The listing builds one solid part. Answer for the finished solid, in the listing's coordinates (mm). Face numbers are marked on the shaded views. A direction names the side the tool comes from. Round coordinates to 2 decimals unless told otherwise and drop trailing zeros. Write item = value, one per line.
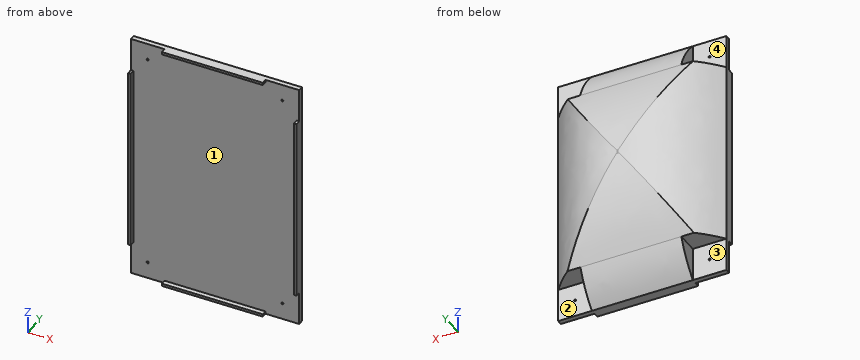
from build123d import *

# Parameters (mm, degrees)
CROQUIS1_W                = 100
CROQUIS1_H                = 150
SALIENTE_EXTRUIR1_DEPTH   = 30
CROQUIS3_W                = 1.5
CROQUIS3_H                = 110
CROQUIS3_W_2              = 60
CROQUIS3_H_2              = 1.5
SALIENTE_EXTRUIR2_DEPTH   = 3
CROQUIS5_W                = 20
CROQUIS5_H                = 20
CORTAR_EXTRUIR2_DEPTH     = 27
CROQUIS6_R                = 0.6
CORTAR_EXTRUIR3_DEPTH     = 95.09569597
SIMETR_A2_COPY_1_SKETCH_R = 0.6
SIMETR_A2_COPY_1_DEPTH    = 95.09569597
CORTAR_EXTRUIR4_DEPTH     = 129.549601322
CORTAR_EXTRUIR5_START     = -150
CORTAR_EXTRUIR5_DEPTH     = 150
CORTAR_EXTRUIR6_DEPTH     = 114.688170172
CORTAR_EXTRUIR7_DEPTH     = 114.688170172


# Read off the part's stored shape, not the designer's step: Cortar-Extruir5
with BuildPart() as part:
    # Croquis1 → Saliente-Extruir1 (new body)
    with BuildSketch(Plane(origin=(0, 0, 0), x_dir=(1, 0, 0), z_dir=(0, 1, 0))):
        Rectangle(CROQUIS1_W, CROQUIS1_H)
    extrude(amount=SALIENTE_EXTRUIR1_DEPTH)

    # Croquis3 → Saliente-Extruir2 (add)
    with BuildSketch(Plane.XZ):
        with Locations((-49.25, 0)):
            Rectangle(CROQUIS3_W, CROQUIS3_H)
        with Locations((0, -74.25)):
            Rectangle(CROQUIS3_W_2, CROQUIS3_H_2)
        with Locations((49.25, 0)):
            Rectangle(CROQUIS3_W, CROQUIS3_H)
        with Locations((0, 74.25)):
            Rectangle(CROQUIS3_W_2, CROQUIS3_H_2)
    extrude(amount=SALIENTE_EXTRUIR2_DEPTH)

    # Croquis5 → Cortar-Extruir2 (cut)
    with BuildSketch(Plane(origin=(0, 30, 0), x_dir=(1, 0, 0), z_dir=(0, 1, 0))):
        with Locations((-40, 65)):
            Rectangle(CROQUIS5_W, CROQUIS5_H)
        with Locations((40, 65)):
            Rectangle(CROQUIS5_W, CROQUIS5_H)
        with Locations((40, -65)):
            Rectangle(CROQUIS5_W, CROQUIS5_H)
        with Locations((-40, -65)):
            Rectangle(CROQUIS5_W, CROQUIS5_H)
    extrude(amount=-CORTAR_EXTRUIR2_DEPTH, mode=Mode.SUBTRACT)

    # Croquis6 → Cortar-Extruir3 (cut, through all)
    with BuildSketch(Plane(origin=(0, 3, 0), x_dir=(1, 0, 0), z_dir=(0, 1, 0))):
        with Locations(Location((40, 65, 0), (0, 0, 270))):
            Circle(CROQUIS6_R)
    cortar_extruir3 = extrude(amount=-CORTAR_EXTRUIR3_DEPTH, mode=Mode.SUBTRACT)

    # Simetría1: Cortar-Extruir3 across plane
    add(cortar_extruir3.mirror(Plane.XY), mode=Mode.SUBTRACT)

    # Simetría2: Cortar-Extruir3 across plane
    add(cortar_extruir3.mirror(Plane(origin=(0, 0, 0), x_dir=(0, 0, 1), z_dir=(1, 0, 0))), mode=Mode.SUBTRACT)

    # Simetría2 copy 1 sketch → Simetría2 copy 1 (cut, through all)
    with BuildSketch(Plane(origin=(0, 3, 0), x_dir=(-1, 0, 0), z_dir=(0, 1, 0))):
        with Locations(Location((40, 65, 0), (0, 0, 270))):
            Circle(SIMETR_A2_COPY_1_SKETCH_R)
    extrude(amount=-SIMETR_A2_COPY_1_DEPTH, mode=Mode.SUBTRACT)

    # Croquis7 → Cortar-Extruir4 (cut, through all)
    with BuildSketch(Plane.ZY.offset(50)):
        with BuildLine():
            Line((-55, 30), (-55, 15.839120061))
            add(Edge.make_bspline(
                [(-55, 15.839120061), (-28.872240535, 29.681618902), (-0.383648773, 29.996375418)],
                knots=[0.272557177, 0.272557177, 0.272557177, 0.972153635, 0.972153635, 0.972153635], degree=2))
            add(Edge.make_bspline(
                [(-0.015370594, 30), (-0.199457484, 29.998481088), (-0.383648773, 29.996375418)],
                knots=[0.9954153, 0.9954153, 0.9954153, 1, 1, 1], degree=2))
            Line((-0.015370594, 30), (-55, 30))
        make_face()
        with BuildLine():
            Line((55, 30), (1.887981045, 30))
            add(Edge.make_bspline(
                [(55, 16.129627481), (29.637077968, 29.770366226), (1.887981045, 30)],
                knots=[0.278550096, 0.278550096, 0.278550096, 0.971678885, 0.971678885, 0.971678885], degree=2))
            Line((55, 16.129627481), (55, 30))
        make_face()
    extrude(amount=-CORTAR_EXTRUIR4_DEPTH, mode=Mode.SUBTRACT)

    # Cortar-Extruir5 outline → Cortar-Extruir5 (cut)
    with BuildSketch(Plane.XY.offset(75).offset(CORTAR_EXTRUIR5_START)):
        with BuildLine():
            Line((7.5e-08, 30.000000001), (-50, 30))
            Line((-50, 30), (-50, 3))
            add(Edge.make_bspline(
                [(-50, 3), (-28.36157969, 29.799939616), (7.5e-08, 30.000000001)],
                knots=[0, 0, 0, 0.985180711, 0.985180711, 0.985180711], degree=2))
        make_face()
        with BuildLine():
            Line((50, 3), (50, 30))
            Line((50, 30), (0.854762637, 30))
            add(Edge.make_bspline(
                [(0.854762637, 30), (28.715142785, 29.789747772), (50, 3)],
                knots=[0.41802479, 0.41802479, 0.41802479, 1.368246178, 1.368246178, 1.368246178], degree=2))
        make_face()
    extrude(amount=CORTAR_EXTRUIR5_DEPTH, mode=Mode.SUBTRACT)

    # Croquis10 → Cortar-Extruir6 (cut, through all)
    with BuildSketch(Plane.ZY.offset(30)):
        with BuildLine():
            Line((75, 3), (75, 42.786726144))
            Line((75, 42.786726144), (55, 42.786726144))
            Line((55, 42.786726144), (55, 16.107425877))
            add(Edge.make_bspline(
                [(75, 3), (66.353698685, 12.015089749), (55, 16.107425877)],
                knots=[0, 0, 0, 1, 1, 1], degree=2))
        make_face()
    extrude(amount=-CORTAR_EXTRUIR6_DEPTH, mode=Mode.SUBTRACT)

    # Croquis11 → Cortar-Extruir7 (cut, through all)
    with BuildSketch(Plane.ZY.offset(30)):
        with BuildLine():
            Line((-75, 3), (-75, 36.400642598))
            Line((-75, 36.400642598), (-55, 36.400642598))
            Line((-55, 36.400642598), (-55, 15.839120066))
            add(Edge.make_bspline(
                [(-75, 3), (-66.12999018, 11.527113216), (-55, 15.839120066)],
                knots=[0, 0, 0, 1, 1, 1], degree=2))
        make_face()
    extrude(amount=-CORTAR_EXTRUIR7_DEPTH, mode=Mode.SUBTRACT)


solid = part.part
Q1. Find the intervals of material crossed by line 1 (X direction, y = 1.1, z = 65); line 2 (Z direction, x = 40, y = 1); line 3 (X direction, y = -1, z = -33), in increasing order. Write a range as from..to.
Model answer:
line_1 = -50..-40.6, -39.4..39.4, 40.6..50
line_2 = -75..-65.6, -64.4..64.4, 65.6..75
line_3 = -50..-48.5, 48.5..50
Q2. For the marked faces 3 and 4, determine the directions among +Z, -Z, +X, -X, +Y, -Y from which every point of the face is accessible in a straight line to the end or side of a thin tool.
Model answer:
face_3 = -Z, -X, +Y
face_4 = +Z, -X, +Y
Q3. Flat-ended cylindrical pins translate along their axes: P1, Ø22, axis at x = 39, z = 60.5, coming from the +Y side; P2, Ø10.5, axis at y = 10, z = 61, coming from the +X side; P3, Ø14, axis at y = 12, z = -69, coming from the -X side. Find the tip coordinate at first contact, or state that the pin passes through.
Model answer:
P1 = 18.43
P2 = 30
P3 = -30
Q4. Determine the mould class of the marked faces 1 and 2 for opening direction X: released by +X, released by -X, zero draft, split by the parting line, or undercut.
Model answer:
face_1 = undercut
face_2 = zero draft
